Input: part model. Units: mm. Frame: model coordinates. Coordinates: 2 decimals unless noted, no trailing zeros. Loops run counter-clockwise (first coordinate to the right, second up) from the corner with the lowest first, then second, coordinate; pieces in that order, holes last.
Item 1: Section A-A on y = 20. Return loops of the section in (x, z).
Item 2: Contact query for a flat-ended pin moving along its axis: P1, Ø6.5, axis at x = 138, y = 20, coming from the -Z side. Output: stop coordinate, or through.
Item 3: Ray query, line 1 along X through (y, z) = (20, 2); line 2 along Y through (x, z) = (162, 2.1); line 3 along Y through (x, z) = (45.5, 0.55). Return the intervals inside material, ascending.
Item 4: Section B-B on x = 138. Return loops of the section in (y, z), and give its area (3 significant figures).
Item 5: Section C-C on z = 2.05. Return loops of the section in (x, y).
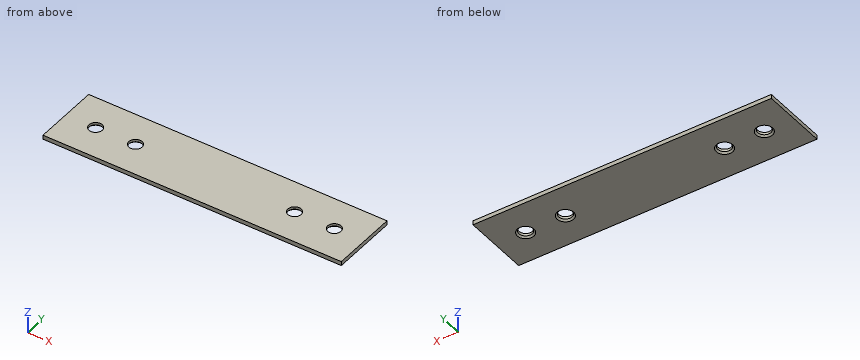
Autodesk Inventor part; units mm, degrees
ref_plane "YZ Plane" through (0, 0, 0) normal (1, 0, 0) x (0, 1, 0)
ref_plane "XZ Plane" through (0, 0, 0) normal (0, 1, 0) x (-1, 0, 0)
ref_plane "XY Plane" through (0, 0, 0) normal (0, 0, 1) x (1, 0, 0)
sketch "Szkic1" plane through (0, 0, 0) normal (0, 0, 1) x (1, 0, 0)
  line L0 (0, 0) -> (180, 0)
  line L1 (180, 0) -> (180, 40)
  line L2 (180, 40) -> (0, 40)
  line L3 (0, 40) -> (0, 0)
  line L4 (0, 20) -> (180, 20) construction
  line L5 (90, 0) -> (90, 40) construction
  line L6 (45, 0) -> (45, 40) construction
  line L7 (18, 40) -> (18, 0) construction
  circle A0 centre (18, 20) radius 4
  line L8 (30, 40) -> (30, 0) construction
  circle A1 centre (42, 20) radius 4
  circle A2 centre (162, 20) radius 4
  circle A3 centre (138, 20) radius 4
  dimension "d0" = 180
  dimension "d1" = 40
  dimension "d2" = 45
  dimension "d3" = 18
  dimension "d5" = 8
  dimension "d6" = 30
extrude "Wyciągnięcie proste1" add sketch "Szkic1" along normal blind 2.5 contours L3 L2 L1 L0 | A0 | A1 | A2 | A3
hole "Otwór2" at (18, 20, 0) at (42, 20, 0) at (138, 20, 0) at (162, 20, 0) direction (0, 0, 1) diameter 8 end through all countersink diameter 10 countersink angle 90
properties part number "lacznik_plaski_180_40_2p5"
Results found:
1. outline: (0, 0) - (13, 0) - (14, 1) - (14, 2.5) - (0, 2.5) - close; (22, 1) - (23, 0) - (37, 0) - (38, 1) - (38, 2.5) - (22, 2.5) - close; (46, 1) - (47, 0) - (133, 0) - (134, 1) - (134, 2.5) - (46, 2.5) - close; (142, 1) - (143, 0) - (157, 0) - (158, 1) - (158, 2.5) - (142, 2.5) - close; (166, 1) - (167, 0) - (180, 0) - (180, 2.5) - (166, 2.5) - close
2. P1: passes through
3. line 1: x = 0 to 14, 22 to 38, 46 to 134, 142 to 158, 166 to 180
3. line 2: y = 0 to 16, 24 to 40
3. line 3: y = 0 to 17.25, 22.75 to 40
4. outline: (0, 0) - (15, 0) - (16, 1) - (16, 2.5) - (0, 2.5) - close; (24, 1) - (25, 0) - (40, 0) - (40, 2.5) - (24, 2.5) - close
4. area: 79.0 mm2
5. outline: (0, 0) - (180, 0) - (180, 40) - (0, 40) - close; hole circle Ø8 at (18, 20); hole circle Ø8 at (42, 20); hole circle Ø8 at (138, 20); hole circle Ø8 at (162, 20)
